```python
from build123d import *

# Parameters (mm, degrees)
SKETCH1_R                 = 5
BOSS_EXTRUDE1_DEPTH       = 3.175
SKETCH4_R                 = 6.35
BIG_INCO_PIN_HOLE_DEPTH   = 4.175
CIRPATTERN3_COUNT         = 16
SKETCH5_R                 = 3.175
SMALL_INCO_PIN_HOLE_DEPTH = 4.175
CIRPATTERN4_COUNT         = 4


with BuildPart() as part:
    # Sketch1 → Boss-Extrude1 (new body)
    with BuildSketch(Plane(origin=(0, 0, 0), x_dir=(1, 0, 0), z_dir=(0, 1, 0))):
        with BuildLine():
            Line((56.288245367, 65.268501488), (36.185821844, 45.166077965))
            ThreePointArc((36.185821844, 45.166077965), (0, 57.8739), (-36.185821844, 45.166077965))
            Line((-36.185821844, 45.166077965), (-56.288245367, 65.268501488))
            Line((-56.288245367, 65.268501488), (-65.268501488, 56.288245367))
            Line((-65.268501488, 56.288245367), (-45.166077965, 36.185821844))
            ThreePointArc((-45.166077965, 36.185821844), (-57.8739, 0), (-45.166077965, -36.185821844))
            Line((-45.166077965, -36.185821844), (-65.268501488, -56.288245367))
            Line((-65.268501488, -56.288245367), (-56.288245367, -65.268501488))
            Line((-56.288245367, -65.268501488), (-36.185821844, -45.166077965))
            ThreePointArc((-36.185821844, -45.166077965), (0, -57.8739), (36.185821844, -45.166077965))
            Line((36.185821844, -45.166077965), (56.288245367, -65.268501488))
            Line((56.288245367, -65.268501488), (65.268501488, -56.288245367))
            Line((65.268501488, -56.288245367), (45.166077965, -36.185821844))
            ThreePointArc((45.166077965, -36.185821844), (57.8739, 0), (45.166077965, 36.185821844))
            Line((45.166077965, 36.185821844), (65.268501488, 56.288245367))
            Line((65.268501488, 56.288245367), (56.288245367, 65.268501488))
        make_face()
        Circle(SKETCH1_R, mode=Mode.SUBTRACT)
    extrude(amount=BOSS_EXTRUDE1_DEPTH)

    # Sketch4 → Big Inco Pin Hole (cut, through all)
    with BuildSketch(Plane(origin=(0, 3.175, 0), x_dir=(1, 0, 0), z_dir=(0, 1, 0))):
        with Locations((46.7614, 0)):
            Circle(SKETCH4_R)
    big_inco_pin_hole = extrude(amount=-BIG_INCO_PIN_HOLE_DEPTH, mode=Mode.SUBTRACT)

    # CirPattern3: Big Inco Pin Hole ×16 about axis
    cirpattern3_axis = Axis((0, 0, 0), (0, 1, 0))
    for i in range(1, CIRPATTERN3_COUNT):
        add(big_inco_pin_hole.rotate(cirpattern3_axis, i * 360 / CIRPATTERN3_COUNT), mode=Mode.SUBTRACT)

    # Sketch5 → Small Inco Pin Hole (cut, through all)
    with BuildSketch(Plane(origin=(0, 3.175, 0), x_dir=(1, 0, 0), z_dir=(0, 1, 0))):
        with Locations((8.980256121, 8.980256121)):
            Circle(SKETCH5_R)
        with Locations((56.288245367, 56.288245367)):
            Circle(SKETCH5_R)
    small_inco_pin_hole = extrude(amount=-SMALL_INCO_PIN_HOLE_DEPTH, mode=Mode.SUBTRACT)

    # CirPattern4: Small Inco Pin Hole ×4 about axis
    cirpattern4_axis = Axis((0, 0, 0), (0, 1, 0))
    for i in range(1, CIRPATTERN4_COUNT):
        add(small_inco_pin_hole.rotate(cirpattern4_axis, i * 360 / CIRPATTERN4_COUNT), mode=Mode.SUBTRACT)


solid = part.part
```
The listing builds one solid part. Answer for the finished solid, in the listing's coordinates (mm). A direction names the side the tool comes from. Coordinates: 2 decimals unless noted, no trailing zeros. Loops run counter-clockwise (first coordinate to the right, second up) from the corner with the lowest first, then second, coordinate; pieces in that order, holes last. Notation, with made-up numbers: (-22.75, 0) - (-14.75, 0) arc R8 ccw to (-14.75, 11) - close; hole circle Ø8 at (-11.75, 57). An arc over 180 degrees is marked (long way). Use a Markdown table: item, result. Add a question column.
1) Given pin 1 (6 mm diameter, centred on x = -47, z = 5, fed in from -Y); pin 2 (1.5 mm diameter, centred on x = -33, y = 0.5, fed in from +Z); pin 3 (1 mm diameter, centred on x = -21.5, y = 2.5, fed in from -Z), each flat-ended and moving along its own axis, determine where each tip first touches the part or whether it passes through.
2) Find the intervals of material crossed by line 1 (X direction, y = 0.95, z = 52.5); line 2 (X direction, y = 2.6, z = 46.5); line 3 (Z direction, x = -40, y = 0.6), in increasing order.
3) The mould has two halves that part along Z. Classify faces 1 (the flat face through (46.1, 1.57, 55.08)), 2 (the flat face through (60.841, 1.565, -60.716)), 3 (the cylindrical face through (10.445, 1.61, -6.163)): released by +Z, released by -Z, zero draft, split by the parting line, or undercut.
4) For faces 4 (the flat face through (-55.36, 1.57, -46.38)), 5 (the flat face through (-46.1, 1.57, -55.08)), 6 (the cylindrical face through (40.418, 1.61, -0.279)), determine the directions among +Z, -Z, +X, -X, +Y, -Y from which every point of the face is accessible in a straight line to the end or side of a thin tool.
5) The part is cut by section C-C, the plane x = 14. Give the vertices of the cut face in (y, z) (3 decimals), and give its area (3 significant figures).
6) The part is cut by section D-D, the plane z = 31. Give the vertices of the cut face in (x, y) (3 decimals), and give its area (3 significant figures).
7) The part is cut by section A-A, the plane z = 0. Give the vertices of the cut face in (x, y) (3 decimals).
8) The part is cut by section B-B, the plane x = 0. Give the vertices of the cut face in (y, z) (3 decimals), and give its area (3 significant figures).
Here are the results:
| question | item | result |
|---|---|---|
| 1 | pin 1 | stops at y = 0 |
| 1 | pin 2 | stops at z = 48.06 |
| 1 | pin 3 | stops at z = -53.93 |
| 2 | line 1 | x = -61.48 to -43.52, -24.35 to -2.72, 2.72 to 24.35, 43.52 to 61.48 |
| 2 | line 2 | x = -55.48 to -37.52, -34.45 to -23.32, -12.47 to -6.34, 6.34 to 12.47, 23.32 to 34.45, 37.52 to 55.48 |
| 2 | line 3 | z = -48.98 to -23.38, -12.41 to 12.41, 23.38 to 48.98 |
| 3 | face 1 | released by +Z |
| 3 | face 2 | released by -Z |
| 3 | face 3 | undercut |
| 4 | face 4 | -X, +Y, -Y |
| 4 | face 5 | -Z, +Y, -Y |
| 4 | face 6 | +Y, -Y |
| 5 | outline | (0, -56.155) - (3.175, -56.155) - (3.175, -48.217) - (0, -48.217) - close; (0, -38.187) - (3.175, -38.187) - (3.175, 38.187) - (0, 38.187) - close; (0, 48.217) - (3.175, 48.217) - (3.175, 56.155) - (0, 56.155) - close |
| 5 | area | 293 mm^2 |
| 6 | outline | (-48.871, 0) - (-39.07, 0) - (-39.07, 3.175) - (-48.871, 3.175) - close; (-27.061, 0) - (27.061, 0) - (27.061, 3.175) - (-27.061, 3.175) - close; (39.07, 0) - (48.871, 0) - (48.871, 3.175) - (39.07, 3.175) - close |
| 6 | area | 234 mm^2 |
| 7 | outline | (-57.874, 0) - (-53.111, 0) - (-53.111, 3.175) - (-57.874, 3.175) - close; (-40.411, 0) - (-5, 0) - (-5, 3.175) - (-40.411, 3.175) - close; (5, 0) - (40.411, 0) - (40.411, 3.175) - (5, 3.175) - close; (53.111, 0) - (57.874, 0) - (57.874, 3.175) - (53.111, 3.175) - close |
| 8 | outline | (0, -57.874) - (3.175, -57.874) - (3.175, -53.111) - (0, -53.111) - close; (0, -40.411) - (3.175, -40.411) - (3.175, -5) - (0, -5) - close; (0, 5) - (3.175, 5) - (3.175, 40.411) - (0, 40.411) - close; (0, 53.111) - (3.175, 53.111) - (3.175, 57.874) - (0, 57.874) - close |
| 8 | area | 255 mm^2 |
